```python
from build123d import *

# Parameters (mm, degrees)
F0_R     = 11.1125
F1_DEPTH = 24.384
F0_W     = 9.652
F0_H     = 9.652
F2_DEPTH = 12.7
F3_R     = 0.381


with BuildPart() as f1:
    # F0 (on Front) → F1 (new body)
    with BuildSketch(Plane.XZ):
        Circle(F0_R)
        with BuildLine():
            ThreePointArc((3.770104, 6.985), (6.816491, 4.066861), (7.9375, 0))
            ThreePointArc((7.9375, 0), (6.816491, -4.066861), (3.770104, -6.985))
            ThreePointArc((3.770104, -6.985), (0, -7.9375), (-3.770104, -6.985))
            ThreePointArc((-3.770104, -6.985), (-7.9375, 0), (-3.770104, 6.985))
            ThreePointArc((-3.770104, 6.985), (0, 7.9375), (3.770104, 6.985))
        make_face(mode=Mode.SUBTRACT)
        with BuildLine():
            ThreePointArc((-3.770104, -6.985), (0, -7.9375), (3.770104, -6.985))
            Line((3.770104, -6.985), (-3.770104, -6.985))
        make_face()
        with BuildLine():
            Line((-3.770104, 6.985), (3.770104, 6.985))
            ThreePointArc((3.770104, 6.985), (0, 7.9375), (-3.770104, 6.985))
        make_face()
    extrude(amount=F1_DEPTH)

    # F0 (on Front) → F2 (join)
    with BuildSketch(Plane.XZ):
        with BuildLine():
            ThreePointArc((3.770104, -6.985), (6.816491, -4.066861), (7.9375, 0))
            ThreePointArc((7.9375, 0), (6.816491, 4.066861), (3.770104, 6.985))
            Line((3.770104, 6.985), (-3.770104, 6.985))
            ThreePointArc((-3.770104, 6.985), (-7.9375, 0), (-3.770104, -6.985))
            Line((-3.770104, -6.985), (3.770104, -6.985))
        make_face()
        Rectangle(F0_W, F0_H, mode=Mode.SUBTRACT)
    extrude(amount=F2_DEPTH)

    # F3
    f3_edges = [f1.edges().sort_by_distance(p)[0] for p in [
        (-11.1125, -24.384, 0),
        (-11.1125, 0, 0),
    ]]
    fillet(f3_edges, radius=F3_R)


solid = f1.part
```
Part model, mm, in its own coordinate system. A direction names the side the tool comes from. Round coordinates to 2 decimals unless told otherwise and drop trailing zeros. Loops run counter-clockwise (first coordinate to the right, second up) from the corner with the lowest first, then second, coordinate; pieces in that order, holes last.
1. Drill centre lines: line 1 along X through (y, z) = (-19.25, -3.5); line 2 along X through (y, z) = (-12.5, -2); line 3 along Z through (x, y) = (1.25, -14.5) (3 decimals). Where is each one in solid material? Low to high.
Solutions:
line 1: x = -10.55 to -7.12, 7.12 to 10.55
line 2: x = -10.93 to -4.83, 4.83 to 10.93
line 3: z = -11.042 to -6.985, 6.985 to 11.042
2. Flat gauge pins, fed straight in: pin 1 (7 mm diameter, centred on x = -3.5, z = 0.5, fed in from -Y); pin 2 (5 mm diameter, centred on x = -5.5, y = -22, fed in from -Z); pin 3 (2 mm diameter, centred on y = -5.5, z = -5, fed in from -X). Where does each tip first touch, or does it go through?
Solutions:
pin 1: stops at y = -12.7
pin 2: stops at z = -10.7
pin 3: stops at x = -10.37
3. Two-plate mould, pull along Z, no slides. Class faces 4 (the face through (10.6, -12.03, 3.34)), 5 (the face through (-5, -12.7, 0)), 6 (the face through (0, 0, 5)): pulls with the +Z half, pulls with the -Z half, needs draft (parallel to the pull), parting line crosses it, or undercut.
Solutions:
face 4: parting line crosses it
face 5: undercut
face 6: needs draft
4. Slice it at B-B (y = -9.25). Give the cut face in (x, z) (1 decimal), and give its area (3 significant figures).
Solutions:
outline: circle Ø22.2 at (0, 0); hole (-4.8, -4.8) - (4.8, -4.8) - (4.8, 4.8) - (-4.8, 4.8) - close
area: 295 mm2
5. Slice it at C-C (y = -14.25). Give the cut face in (x, z) (1 decimal), and give its area (3 significant figures).
Solutions:
outline: circle Ø22.2 at (0, 0); hole (-3.8, -7) - (3.8, -7) arc R7.9 ccw to (3.8, 7) - (-3.8, 7) arc R7.9 ccw to start
area: 200 mm2
6. 3-axis set-ups, long thin cutter, end or side, ignore diameter. For faces 1 (the face through (0, -18, -6.985)), 2 (the face through (-0.2, -24.384, 7.3)), 3 (the face through (-4.826, -6, 0)): which of +Z, -Z, +X, -X, +Y, -Y reach the whole face in a straight line?
Solutions:
face 1: -Y
face 2: +Z, -Z, +X, -X, -Y
face 3: +Y, -Y
7. Slice it at A-A (x = 0). Give the cut face in (y, z) (1 decimal), and give its area (3 significant figures).
Solutions:
outline: (-24.4, -10.7) arc R0.4 ccw to (-24, -11.1) - (-0.4, -11.1) arc R0.4 ccw to (0, -10.7) - (0, -4.8) - (-12.7, -4.8) - (-12.7, -7) - (-24.4, -7) - close; (-24.4, 7) - (-12.7, 7) - (-12.7, 4.8) - (0, 4.8) - (0, 10.7) arc R0.4 ccw to (-0.4, 11.1) - (-24, 11.1) arc R0.4 ccw to (-24.4, 10.7) - close
area: 256 mm2
